from build123d import *

# Parameters (mm, degrees)
F0_R     = 6
F0_R_2   = 5.236084
F1_DEPTH = 10
F2_R     = 10
F3_DEPTH = 8


with BuildPart() as f1:
    # F0 (on Top) → F1 (new body)
    with BuildSketch(Plane.XY):
        with BuildLine():
            ThreePointArc((4.789302, -36.367918), (21.195339, -23.224109), (41.554008, -17.985565))
            ThreePointArc((41.554008, -17.985565), (58.833284, 0), (41.554008, 17.985565))
            ThreePointArc((41.554008, 17.985565), (21.195339, 23.224109), (4.789302, 36.367918))
            ThreePointArc((4.789302, 36.367918), (-15.199612, 41.958896), (-27.166716, 25))
            Line((-27.166716, 25), (-27.166716, -25))
            ThreePointArc((-27.166716, -25), (-15.199612, -41.958896), (4.789302, -36.367918))
        make_face()
        with Locations((-9.166716, -25)):
            Circle(F0_R, mode=Mode.SUBTRACT)
        with Locations((-9.166716, 25)):
            Circle(F0_R, mode=Mode.SUBTRACT)
        with Locations((40.833284, 0)):
            Circle(F0_R_2, mode=Mode.SUBTRACT)
    extrude(amount=F1_DEPTH)

    # F2 (on Front) → F3 (join, symmetric)
    with BuildSketch(Plane.XZ):
        with BuildLine():
            ThreePointArc((-55.095504, 38.911565), (-89.855534, 29.481496), (-69.166716, 0))
            Line((-69.166716, 0), (-27.166716, 0))
            Line((-27.166716, 0), (0, 0))
            Line((0, 0), (24.854559, 0))
            Line((24.854559, 0), (24.854559, 10))
            ThreePointArc((24.854559, 10), (-17.653944, 17.449895), (-55.095504, 38.911565))
        make_face()
        with Locations((-69.166716, 22)):
            Circle(F2_R, mode=Mode.SUBTRACT)
    extrude(amount=F3_DEPTH, both=True)


solid = f1.part
Part model, mm, in its own coordinate system. A direction names the side the tool comes from. Give positions to 0.01 mm unless a question says otherwise; leave off trailing zeros. Loops run counter-clockwise (first coordinate to the right, second up) from the corner with the lowest first, then second, coordinate; pieces in that order, holes last. Notation, with made-up numbers: M 45,-38 L 53,-38 A16 cw 53,-22 Z; hole C 19,-22.5 d9. An arc over 180 degrees is marked long. Put each result on its own line as item: value. Start each with the question number.
1) Flat gauge pins, fed straight in: pin 1 (3 mm diameter, centred on y = 19.5, z = 5, fed in from -X); pin 2 (23 mm diameter, centred on x = -69.17, z = 22, fed in from -Y); pin 3 (3 mm diameter, centred on y = -4, z = 7.5, fed in from +X); pin 4 (9.5 mm diameter, centred on x = -9.17, y = 25, fed in from -Z). Where does each tip first touch, or does it go through?
2) Saw through at A-A (y = 0). List the corners of the cut face in (x, z), then the cut area to 3 significant figures.
3) Saw through at C-C (z = 30). List the corners of the cut face in (x, y).
4) 3-axis set-ups, long thin cutter, end or side, ignore diameter. For faces 1 (the cylindrical face through (-14.91, 42.06, 4.93)), 2 (the flat face through (-27.167, 17, 5)): which of +Z, -Z, +X, -X, +Y, -Y reach the whole face in a straight line?
5) Saw through at B-B (x = -6). List the corners of the cut face in (y, z).
6) Probe probe 1 along Y at (x, z) = (-12, 6.5); probe 2 along Z at (x, y) = (-19.5, 33); probe 3 along Y at (x, z) = (-30, 11). List the from-to ranges inside material, lowest first.
7) Pull direction X, two halves, no side cores. Call faces 3 (the flat face through (-27.167, -16, 5)), 4 (the cylindrical face through (-89.65, -0.11, 30.03)), 5 (the cylindrical face through (-59.628, 0.112, 25.004)): +X half, -X half, draft (parallel to the pull), parting line (faces both ways), or undercut.
8) Saw through at D-D (y = -29.5). List the corners of the cut face in (x, z), then the cut area to 3 significant figures.
Numbers:
1. pin 1: x = -27.17
1. pin 2: y = -8
1. pin 3: x = 58.66
1. pin 4: through
2. outline: M -69.17,0 L 35.6,0 L 35.6,10 L 24.85,10 A125 cw -55.1,38.91 A22 ccw long Z; M 46.07,0 L 58.83,0 L 58.83,10 L 46.07,10 Z; hole C -69.17,22 d20
2. area: 2,810 mm^2
3. outline: M -89.66,-8 L -75.17,-8 L -75.17,8 L -89.66,8 Z; M -63.17,-8 L -42.97,-8 L -42.97,8 L -63.17,8 Z
4. face 1: +Z, -Z, +Y
4. face 2: +Z, -Z, -X, +Y
5. outline: M -42.72,0 L -30.1,0 L -30.1,10 L -42.72,10 Z; M -19.9,0 L 19.9,0 L 19.9,10 L 8,10 L 8,13.87 L -8,13.87 L -8,10 L -19.9,10 Z; M 30.1,0 L 42.72,0 L 42.72,10 L 30.1,10 Z
6. probe 1: -42.78 to -30.29, -19.71 to 19.71, 30.29 to 42.78
6. probe 2: 0 to 10
6. probe 3: -8 to 8
7. face 3: -X half
7. face 4: parting line
7. face 5: undercut
8. outline: M -26.6,0 L -13.14,0 L -13.14,10 L -26.6,10 Z; M -5.2,0 L 11.59,0 L 11.59,10 L -5.2,10 Z
8. area: 302 mm^2
